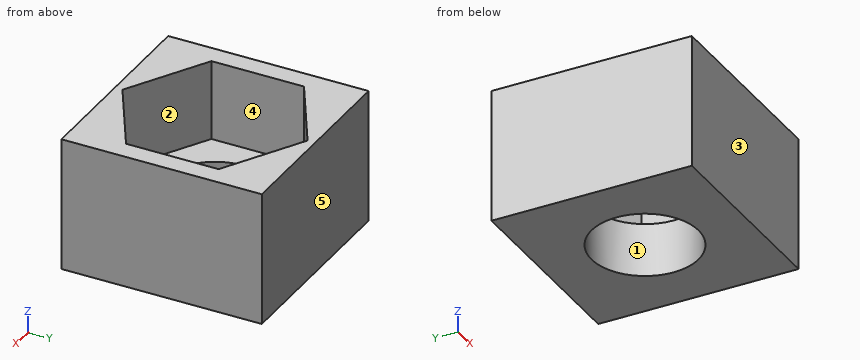
```python
from build123d import *

# Parameters (mm, degrees)
F0_W     = 15
F0_H     = 15
F1_DEPTH = 10
F3_DEPTH = 6
F4_R     = 4
F5_DEPTH = 25


with BuildPart() as f1:
    # F0 (on Top) → F1 (new body)
    with BuildSketch(Plane.XY):
        Rectangle(F0_W, F0_H)
    extrude(amount=F1_DEPTH)

    # F2 (on face) → F3 (cut)
    with BuildSketch(Plane.XY.offset(10)):
        Polygon((0, -6.928203), (6, -3.464102), (6, 3.464102), (0, 6.928203), (-6, 3.464102), (-6, -3.464102), align=None)
    extrude(amount=-F3_DEPTH, mode=Mode.SUBTRACT)

    # F4 (on face) → F5 (cut)
    with BuildSketch(Plane.XY.offset(4)):
        Circle(F4_R)
    extrude(amount=-F5_DEPTH, mode=Mode.SUBTRACT)


solid = f1.part
```
Here's how the part is built. I have some questions about the finished solid (model axes, mm). Face numbers are marked on the shaded views. A direction names the side the tool comes from. Coordinates: 2 decimals unless noted, no trailing zeros. Write each loop counter-clockwise with the first axis right and the second up, starting at its lowest first coordinate (ties: lowest second). Pieces come first, ordered by that corner, then holes. Notation, with made-up numbers: (14, -38.75) -> (52, -38.75) arc R36 ccw to (52, -1.75) -> close; hole circle Ø11 at (-7.5, 83). An arc over 180 degrees is marked (long way). Use a Markdown table: item, result. Add a question column.
(1) For the marked faces 1 and 2, which set-ups out of +Z, -Z, +X, -X, +Y, -Y let a thin tool reach every point of the face, with its end or its side?
(2) We'd pull the mould along Y, two halves only. Please class the marked faces 3, 4 and 5: +Y half, -Y half, draft (parallel to the pull), parting line (faces both ways), or undercut.
(3) If we section it at A-A, the plane y = 0: Write out the boundary of the cut face in (x, z).
(4) If we section it at C-C, the plane x = 1.75: Write out the boundary of the cut face in (y, z), and give its area (3 significant figures).
(5) If we section it at D-D, the plane y = 4.5: Write out the boundary of the cut face in (x, z), and give its area (3 significant figures).
(6) If we section it at B-B, the plane z = 8.75: Write out the boundary of the cut face in (x, y).
(7) Please list where these lines run through material, in increasing order: line 1 (Y direction, x = 0, z = 2.8); line 2 (Y direction, x = -1.5, z = 1.75); line 3 (X direction, y = 2.5, z = 3).
Outcome:
| question | item | result |
|---|---|---|
| 1 | face 1 | +Z, -Z |
| 1 | face 2 | +Z |
| 2 | face 3 | -Y half |
| 2 | face 4 | undercut |
| 2 | face 5 | +Y half |
| 3 | outline | (-7.5, 0) -> (-4, 0) -> (-4, 4) -> (-6, 4) -> (-6, 10) -> (-7.5, 10) -> close; (4, 0) -> (7.5, 0) -> (7.5, 10) -> (6, 10) -> (6, 4) -> (4, 4) -> close |
| 4 | outline | (-7.5, 0) -> (-3.6, 0) -> (-3.6, 4) -> (-5.92, 4) -> (-5.92, 10) -> (-7.5, 10) -> close; (3.6, 0) -> (7.5, 0) -> (7.5, 10) -> (5.92, 10) -> (5.92, 4) -> (3.6, 4) -> close |
| 4 | area | 50.2 mm^2 |
| 5 | outline | (-7.5, 0) -> (7.5, 0) -> (7.5, 10) -> (4.21, 10) -> (4.21, 4) -> (-4.21, 4) -> (-4.21, 10) -> (-7.5, 10) -> close |
| 5 | area | 99.5 mm^2 |
| 6 | outline | (-7.5, -7.5) -> (7.5, -7.5) -> (7.5, 7.5) -> (-7.5, 7.5) -> close; hole (-6, -3.46) -> (0, -6.93) -> (6, -3.46) -> (6, 3.46) -> (0, 6.93) -> (-6, 3.46) -> close |
| 7 | line 1 | y = -7.5 to -4, 4 to 7.5 |
| 7 | line 2 | y = -7.5 to -3.71, 3.71 to 7.5 |
| 7 | line 3 | x = -7.5 to -3.12, 3.12 to 7.5 |
